Geometry: final body of the model. Coordinates: model frame, mm. A direction names the side the tool comes from. Give positions to 0.01 mm unless a question says otherwise; leave off trailing zeros. Write each loop counter-clockwise with the first axis right and the second up, starting at its lowest first coordinate (ties: lowest second). Pieces come first, ordered by that corner, then holes. Notation, with made-up numbers: (38.25, 65) -> (48.25, 65) arc R15 ccw to (48.25, 91) -> close; hole circle Ø6 at (-0.75, -17.75). An arc over 180 degrees is marked (long way). Answer as a JSON object with one key per item and string values. Group by question number.
(1) Section query B-B on x = -18. Output: boundary loops of the cut face in (y, z).
(2) Set-up query: faces 1 (the face through (29.22, 1.06, -27.67)), 2 (the face through (-50.699, 1.06, -48.695)). Return all of +Z, -Z, +X, -X, +Y, -Y with unobstructed straight access to the full face (end or side cutting, diameter ignored); none if empty.
(3) Section query C-C on y = 0.5. State how many separate pieces and enclosed holes the cut face has, plus the area to 3 significant figures.
(4) Material intervals for probe 1 along X at (y, z) = (1.6, 35) (3 decimals); probe 2 along Z at (x, y) = (-47.5, 1.2) (3 decimals); probe 3 along X at (y, z) = (0.95, 44) (3 decimals), sorted ascending.
(5) Section query A-A on z = -15. Output: boundary loops of the cut face in (x, y) (3 decimals), plus the area to 3 significant figures.
(6) Section query D-D on x = -35. Output: boundary loops of the cut face in (y, z).
(7) Draft query along Z for faces 3 (the face through (-29.22, 1.06, 27.67)), 4 (the face through (50.77, 1.06, -48.624)), 5 (the face through (34.54, 1.06, 31.53)), 6 (the face through (-50.77, 1.06, 48.624)). Return one class per face: +Z half, -Z half, draft (parallel to the pull), parting line (faces both ways), or undercut.
from build123d import *

# Parameters (mm, degrees)
SKETCH2_R           = 2
SKETCH2_R_2         = 3.5
BOSS_EXTRUDE1_DEPTH = 2.15


with BuildPart() as part:
    # Sketch2 → Boss-Extrude1 (new body)
    with BuildSketch(Plane(origin=(0, 0, 0), x_dir=(1, 0, 0), z_dir=(0, 1, 0))):
        with BuildLine():
            Line((-52.075, 45.425), (-52.075, -45.425))
            ThreePointArc((-52.075, -45.425), (-50.735013524, -48.660013524), (-47.5, -50))
            Line((-47.5, -50), (47.5, -50))
            ThreePointArc((47.5, -50), (50.735013524, -48.660013524), (52.075, -45.425))
            Line((52.075, -45.425), (52.075, 45.425))
            ThreePointArc((52.075, 45.425), (50.735013524, 48.660013524), (47.5, 50))
            Line((47.5, 50), (-47.5, 50))
            ThreePointArc((-47.5, 50), (-50.735013524, 48.660013524), (-52.075, 45.425))
        make_face()
        with Locations((47.5, -45.425)):
            Circle(SKETCH2_R, mode=Mode.SUBTRACT)
        with Locations((-47.5, -45.425)):
            Circle(SKETCH2_R, mode=Mode.SUBTRACT)
        with Locations((-35, 35)):
            Circle(SKETCH2_R_2, mode=Mode.SUBTRACT)
        with Locations((35, 35)):
            Circle(SKETCH2_R_2, mode=Mode.SUBTRACT)
        with Locations((35, -35)):
            Circle(SKETCH2_R_2, mode=Mode.SUBTRACT)
        with Locations((-35, -35)):
            Circle(SKETCH2_R_2, mode=Mode.SUBTRACT)
        with BuildLine():
            Line((-49, 45.225), (-49, 45.625))
            ThreePointArc((-49, 45.625), (-47.5, 47.125), (-46, 45.625))
            Line((-46, 45.625), (-46, 45.225))
            ThreePointArc((-46, 45.225), (-47.5, 43.725), (-49, 45.225))
        make_face(mode=Mode.SUBTRACT)
        with BuildLine():
            Line((46, 45.225), (46, 45.625))
            ThreePointArc((46, 45.625), (47.5, 47.125), (49, 45.625))
            Line((49, 45.625), (49, 45.225))
            ThreePointArc((49, 45.225), (47.5, 43.725), (46, 45.225))
        make_face(mode=Mode.SUBTRACT)
        with BuildLine():
            Line((-22.075, -30.673828947), (22.075, -30.673828947))
            ThreePointArc((22.075, -30.673828947), (29.146067812, -27.744896759), (32.075, -20.673828947))
            Line((32.075, -20.673828947), (32.075, 20.673828947))
            ThreePointArc((32.075, 20.673828947), (29.146067812, 27.744896759), (22.075, 30.673828947))
            Line((22.075, 30.673828947), (-22.075, 30.673828947))
            ThreePointArc((-22.075, 30.673828947), (-29.146067812, 27.744896759), (-32.075, 20.673828947))
            Line((-32.075, 20.673828947), (-32.075, -20.673828947))
            ThreePointArc((-32.075, -20.673828947), (-29.146067812, -27.744896759), (-22.075, -30.673828947))
        make_face(mode=Mode.SUBTRACT)
    extrude(amount=BOSS_EXTRUDE1_DEPTH)


solid = part.part
Answer list:
{
 "1": {"outline": "(0, -50) -> (2.15, -50) -> (2.15, -30.67) -> (0, -30.67) -> close; (0, 30.67) -> (2.15, 30.67) -> (2.15, 50) -> (0, 50) -> close"},
 "2": {"face 1": "+Y, -Y", "face 2": "-Z, -X, +Y, -Y"},
 "3": {"separate pieces": "1", "enclosed holes": "9", "area": "6,350 mm2"},
 "4": {"probe 1": "-52.075 to -38.5, -31.5 to 31.5, 38.5 to 52.075", "probe 2": "-50 to -47.125, -43.725 to 43.425, 47.425 to 50", "probe 3": "-52.075 to -48.903, -46.097 to 46.097, 48.903 to 52.075"},
 "5": {"outline": "(-52.075, 0) -> (-32.075, 0) -> (-32.075, 2.15) -> (-52.075, 2.15) -> close; (32.075, 0) -> (52.075, 0) -> (52.075, 2.15) -> (32.075, 2.15) -> close", "area": "86.0 mm2"},
 "6": {"outline": "(0, -50) -> (2.15, -50) -> (2.15, -38.5) -> (0, -38.5) -> close; (0, -31.5) -> (2.15, -31.5) -> (2.15, 31.5) -> (0, 31.5) -> close; (0, 38.5) -> (2.15, 38.5) -> (2.15, 50) -> (0, 50) -> close"},
 "7": {"face 3": "undercut", "face 4": "-Z half", "face 5": "undercut", "face 6": "+Z half"}
}
